from build123d import *

# Parameters (mm, degrees)
CUT_EXTRUDE5_START = -20
CUT_EXTRUDE5_DEPTH = 20
FILLET4_R          = 2.5
CUT_EXTRUDE6_START = -86.02405492
SKETCH7_R          = 1.984375
CUT_EXTRUDE6_DEPTH = 143.469271841
CIRPATTERN2_COUNT  = 6


with BuildPart() as part:
    # Sketch1 → Revolve1 (revolve)
    with BuildSketch(Plane(origin=(0, 0, 0), x_dir=(0, 0, -1), z_dir=(1, 0, 0)), mode=Mode.PRIVATE) as revolve1_sk:
        Polygon((-22.6695, -31.75), (-22.6695, 0), (-33, 0), (-33, -24.619433914), (-25.8445, -31.75), align=None)
    revolve(revolve1_sk.sketch.rotate(Axis((0, 0, 0), (0, 1, 0)), 180), axis=Axis((0, 0, 0), (0, 1, 0)))

    # Sketch4 → Cut-Extrude5 (cut)
    with BuildSketch(Plane(origin=(0, 0, 0), x_dir=(1, 0, 0), z_dir=(0, 1, 0)).offset(CUT_EXTRUDE5_START)):
        with BuildLine():
            ThreePointArc((33, 0), (28.578838325, 16.5), (16.5, 28.578838325))
            Line((16.5, 28.578838325), (33, 0))
        make_face()
        with BuildLine():
            Line((-16.5, 28.578838325), (16.5, 28.578838325))
            ThreePointArc((16.5, 28.578838325), (0, 33), (-16.5, 28.578838325))
        make_face()
        with BuildLine():
            Line((-33, 0), (-16.5, 28.578838325))
            ThreePointArc((-16.5, 28.578838325), (-28.578838325, 16.5), (-33, 0))
        make_face()
        with BuildLine():
            ThreePointArc((16.5, -28.578838325), (28.578838325, -16.5), (33, 0))
            Line((33, 0), (16.5, -28.578838325))
        make_face()
        with BuildLine():
            Line((-16.5, -28.578838325), (-33, 0))
            ThreePointArc((-33, 0), (-28.578838325, -16.5), (-16.5, -28.578838325))
        make_face()
        with BuildLine():
            ThreePointArc((-16.5, -28.578838325), (0, -33), (16.5, -28.578838325))
            Line((16.5, -28.578838325), (-16.5, -28.578838325))
        make_face()
    extrude(amount=CUT_EXTRUDE5_DEPTH, mode=Mode.SUBTRACT)

    # Fillet4
    fillet4_edges = [part.edges().sort_by_distance(p)[0] for p in [
        (33, -10, 0),
        (16.5, -10, -28.578838325),
        (-33, -10, 0),
        (16.5, -10, 28.578838325),
        (-16.5, -10, -28.578838325),
        (-16.5, -10, 28.578838325),
    ]]
    fillet(fillet4_edges, radius=FILLET4_R)

    # Sketch7 → Cut-Extrude6 (cut)
    with BuildSketch(Plane.XY.offset(CUT_EXTRUDE6_START)):
        Circle(SKETCH7_R)
    cut_extrude6 = extrude(amount=CUT_EXTRUDE6_DEPTH, mode=Mode.SUBTRACT)

    # CirPattern2: Cut-Extrude6 ×6 about axis
    cirpattern2_axis = Axis((0, 0, 0), (0, -1, 0))
    for i in range(1, CIRPATTERN2_COUNT):
        add(cut_extrude6.rotate(cirpattern2_axis, i * 360 / CIRPATTERN2_COUNT), mode=Mode.SUBTRACT)


solid = part.part
Input: part model. Units: mm. Frame: model coordinates. A direction names the side the tool comes from. Give positions to 0.01 mm unless a question says otherwise; leave off trailing zeros. Order: outer loops, then holes, each group sorted by start corner. A loop starts at its lowest first (then second) coordinate and runs counter-clockwise, first axis right, second up. Notation, with made-up numbers: M 78,1 L 102,1 A25 ccw 102,14 Z; hole C 48,23.5 d2. An arc over 180 degrees is marked long. Answer as a JSON object with one key per item and string values.
1. Cut plane D-D, the plane y = -26. Output: boundary loops of the cut face in (x, z), and give its area (3 significant figures).
Result sheet:
{"outline": "C 0,0 d63.23; hole C 0,0 d45.34", "area": "1,530 mm²"}
2. Pull-direction query (Z, two-part tool) for faces 4 (the flat face through (0, -20, 29)), 5 (the cylindrical face through (32.613, -9.86, 0.018)), 6 (the cylindrical face through (22.212, -1.984, 12.774)); classes: +Z half, -Z half, draft (parallel to the pull), parting line (faces both ways), or undercut.
Result sheet:
{"face 4": "draft", "face 5": "parting line", "face 6": "undercut"}
3. Cut plane A-A, the plane z = 0. Output: boundary loops of the cut face in (x, y), and give its area (3 significant figures).
Result sheet:
{"outline": "M -33,-24.62 L -25.84,-31.75 L -22.67,-31.75 L -22.67,0 L -32.61,0 L -32.61,-20 L -33,-20 Z; M 22.67,-31.75 L 25.84,-31.75 L 33,-24.62 L 33,-20 L 32.61,-20 L 32.61,0 L 22.67,0 Z", "area": "589 mm²"}
4. Reachability of faces 1 (the flat face through (0, -10, -28.579)), 2 (the flat face through (-24.645, -10.14, 14.472)), 3 (the flat face through (24.645, -10.14, -14.472)) from +Z, -Z, +X, -X, +Y, -Y: full face, straight path, thin tool, end or side. Return the list, or none.
Result sheet:
{"face 1": "-Z, +X, -X, +Y", "face 2": "+Z, -X, +Y", "face 3": "-Z, +X, +Y"}
5. Cut plane C-C, the plane y = -15. Output: boundary loops of the cut face in (x, z).
Result sheet:
{"outline": "M -32.28,-1.25 L -17.22,-27.33 A2.5 ccw -15.06,-28.58 L 15.06,-28.58 A2.5 ccw 17.22,-27.33 L 32.28,-1.25 A2.5 ccw 32.28,1.25 L 17.22,27.33 A2.5 ccw 15.06,28.58 L -15.06,28.58 A2.5 ccw -17.22,27.33 L -32.28,1.25 A2.5 ccw Z; hole C 0,0 d45.34"}
6. First-contact query: P1, Ø1, axis at x = 6.5, y = -24, coming from the -Z side; P2, Ø1, axis at y = -19, z = 15, coming from the -X side; P3, Ø1, axis at x = -22, y = -19, coming from the +Z side. Flat tips, straight axial feed; report the tip coordinate or a pass-through.
Result sheet:
{"P1": "z = -32.45", "P2": "x = -24.63", "P3": "z = 19.92"}
7. Cut plane B-B, the plane x = 0. Output: boundary loops of the cut face in (y, z), and give its area (3 significant figures).
Result sheet:
{"outline": "M -31.75,-25.84 L -24.62,-33 L -20,-33 L -20,-28.58 L -1.98,-28.58 L -1.98,-22.67 L -31.75,-22.67 Z; M -31.75,22.67 L -1.98,22.67 L -1.98,28.58 L -20,28.58 L -20,33 L -24.62,33 L -31.75,25.84 Z", "area": "405 mm²"}
8. Ray query, line 1 (Z direction, x = 2, y = -9); line 2 (X direction, y = -16, z = 0); line 3 (X direction, y = -21.5, z = 0). Return the intervals inside material, ascending. Write a range as [from, to].
Result sheet:
{"line 1": "[-28.58, -22.58], [22.58, 28.58]", "line 2": "[-32.61, -22.67], [22.67, 32.61]", "line 3": "[-33, -22.67], [22.67, 33]"}
